```python
from build123d import *

# Parameters (mm, degrees)
BOSS_EXTRUDE1_DEPTH = 26.5
SKETCH2_R           = 3.9
SKETCH2_R_2         = 1.5
CUT_EXTRUDE1_DEPTH  = 4
SKETCH3_R           = 5
SKETCH3_R_2         = 1.5
CUT_EXTRUDE2_DEPTH  = 4


with BuildPart() as part:
    # Sketch1 → Boss-Extrude1 (new body)
    with BuildSketch(Plane(origin=(0, 0, 0), x_dir=(0, 0, -1), z_dir=(1, 0, 0))):
        Polygon((-3, -3), (29.5, -3), (29.5, 0), (0, 0), (0, 30), (-3, 30), align=None)
    extrude(amount=BOSS_EXTRUDE1_DEPTH)

    # Sketch2 → Cut-Extrude1 (cut, through all)
    with BuildSketch(Plane(origin=(0, 0, 0), x_dir=(-1, 0, 0), z_dir=(0, 0, -1))):
        with Locations((-13.25, 15)):
            Circle(SKETCH2_R)
        with Locations((-4.75, 15)):
            Circle(SKETCH2_R_2)
        with Locations((-21.75, 15)):
            Circle(SKETCH2_R_2)
        with BuildLine():
            ThreePointArc((-26.5, 20), (-23.571067812, 27.071067812), (-16.5, 30))
            Line((-16.5, 30), (-26.5, 30))
            Line((-26.5, 30), (-26.5, 20))
        make_face()
        with BuildLine():
            Line((0, 30), (-10, 30))
            ThreePointArc((-10, 30), (-2.928932188, 27.071067812), (0, 20))
            Line((0, 20), (0, 30))
        make_face()
    extrude(amount=-CUT_EXTRUDE1_DEPTH, mode=Mode.SUBTRACT)

    # Sketch3 → Cut-Extrude2 (cut, through all)
    with BuildSketch(Plane(origin=(0, 0, 0), x_dir=(1, 0, 0), z_dir=(0, 1, 0))):
        with Locations((13.25, 14.75)):
            Circle(SKETCH3_R)
        with Locations((21.25, 21.75)):
            Circle(SKETCH3_R_2)
        with Locations((21.25, 7.75)):
            Circle(SKETCH3_R_2)
        with Locations((5.25, 21.75)):
            Circle(SKETCH3_R_2)
        with Locations((5.25, 7.75)):
            Circle(SKETCH3_R_2)
    extrude(amount=-CUT_EXTRUDE2_DEPTH, mode=Mode.SUBTRACT)


solid = part.part
```
Could you check a few things on this model? Use its own coordinates, in mm. A direction names the side the tool comes from. Coordinates: 2 decimals unless noted, no trailing zeros. Loops run counter-clockwise (first coordinate to the right, second up) from the corner with the lowest first, then second, coordinate; pieces in that order, holes last. Notation, with made-up numbers: M -31,-6 L 5,-6 A34 ccw 5,27 Z; hole C -1,78 d6. An arc over 180 degrees is marked long. Put each result on its own line as item: value. Start each with the question number.
(1) Suppose I cut it at A-A on z = -7.75. Please give me the cut outline in (x, y), then the cut area to 3 significant figures.
(2) Will these pins go through, and if not, where does the flat tip stop? P1, Ø8, axis at x = 13.25, z = -14.75, coming from the +Y side; P2, Ø3, axis at x = 22, z = -2, coming from the +Y side; P3, Ø8, axis at x = 23.5, y = 24, coming from the -Z side.
(3) Suppose I cut it at B-B on x = 13.25. Please give me the cut outline in (y, z), then the cut area to 3 significant figures.
(4) Thinking about a two-plate mould opening in Y: for faces 3 (the face through (16.12, 17.64, 1.48)), 4 (the face through (4.925, -1.479, -6.286)), 5 (the face through (13, -3, -9)), 6 (the face through (3.01, 27.15, 1.48)), which applies, pulls with the +Y half, pulls with the -Y half, needs draft (parallel to the pull), parting line crosses it, or undercut?
(5) Suppose I cut it at C-C on z = -14.75. Please give me the cut outline in (x, y).
(6) For faces 1 (the face through (5.055, -1.479, -23.237)), 2 (the face through (7, 0, -15)), which set-ups out of +Z, -Z, +X, -X, +Y, -Y let a thin tool reach every point of the face, with its end or its side?
(7) I need wall thicknesses on line 1 (Z direction, x = 21.25, y = -0.85); line 2 (Y direction, x = 16, z = -24.5); line 3 (Y direction, x = 13.25, z = 0.8). Which ranges of each line are inside material? Lowest first, please. Write a range as from..to.
(8) Suppose I cut it at D-D on x = 5.25. Please give me the cut outline in (y, z).
Solutions:
1. outline: M 0,-3 L 3.75,-3 L 3.75,0 L 0,0 Z; M 6.75,-3 L 19.75,-3 L 19.75,0 L 6.75,0 Z; M 22.75,-3 L 26.5,-3 L 26.5,0 L 22.75,0 Z
1. area: 61.5 mm2
2. P1: passes through
2. P2: stops at y = 0
2. P3: stops at z = 0
3. outline: M -3,-29.5 L 0,-29.5 L 0,-19.75 L -3,-19.75 Z; M -3,-9.75 L 0,-9.75 L 0,0 L 11.1,0 L 11.1,3 L -3,3 Z; M 18.9,0 L 30,0 L 30,3 L 18.9,3 Z
3. area: 134 mm2
4. face 3: undercut
4. face 4: needs draft
4. face 5: pulls with the -Y half
4. face 6: pulls with the +Y half
5. outline: M 0,-3 L 8.25,-3 L 8.25,0 L 0,0 Z; M 18.25,-3 L 26.5,-3 L 26.5,0 L 18.25,0 Z
6. face 1: +Y, -Y
6. face 2: -Z, +X, -X, +Y
7. line 1: z = -29.5..-23.25, -20.25..-9.25, -6.25..3
7. line 2: y = -3..0
7. line 3: y = -3..11.1, 18.9..30
8. outline: M -3,-29.5 L 0,-29.5 L 0,-23.25 L -3,-23.25 Z; M -3,-20.25 L 0,-20.25 L 0,-9.25 L -3,-9.25 Z; M -3,-6.25 L 0,-6.25 L 0,0 L 13.59,0 L 13.59,3 L -3,3 Z; M 16.41,0 L 28.8,0 L 28.8,3 L 16.41,3 Z
